Here's how the part is built. I have some questions about the finished solid (model axes, mm). A direction names the side the tool comes from. Give positions to 0.01 mm unless a question says otherwise; leave off trailing zeros. Write each loop counter-clockwise with the first axis right and the second up, starting at its lowest first coordinate (ties: lowest second). Pieces come first, ordered by that corner, then holes. Notation, with made-up numbers: (40, 37) -> (66, 37) arc R23 cw to (66, 65) -> close; hole circle Ø8 at (79, 49.25). An arc over 180 degrees is marked (long way). Put each result on its own line as item: value. Start each with the question number.
from build123d import *

# Parameters (mm, degrees)
SKETCH_W     = 5
SKETCH_H     = 80
PAD_DEPTH    = 61
PAD001_DEPTH = 61
SKETCH002_W  = 49
SKETCH002_H  = 101.034886
POCKET_DEPTH = 19


with BuildPart() as part:
    # Sketch (on YZ_Plane of Origin) → Pad (new body)
    with BuildSketch(Plane.YZ):
        with Locations((-2.5, 40)):
            Rectangle(SKETCH_W, SKETCH_H)
    extrude(amount=PAD_DEPTH)

    # Sketch001 (on Face5 of Pad) → Pad001 (join)
    with BuildSketch(Plane(origin=(0, 0, 0), x_dir=(0, -1, 0), z_dir=(-1, 0, 0))):
        Polygon((0, 0), (0, 36), (0, 40), (-19, 40), (-19, 36), (-13, 36), (-13, 0), align=None)
    extrude(amount=-PAD001_DEPTH)

    # Sketch002 (on Face1 of Pad001) → Pocket (cut)
    with BuildSketch(Plane(origin=(0, 0, 0), x_dir=(-1, 0, 0), z_dir=(0, 1, 0))):
        with Locations((-30.493867, 45)):
            Rectangle(SKETCH002_W, SKETCH002_H)
    extrude(amount=POCKET_DEPTH, mode=Mode.SUBTRACT)


solid = part.part
1) I want a section at A-A, the plane y = 14. Write out the boundary of the cut face in (x, z).
2) I want a section at C-C, the plane z = 30.5. Write out the boundary of the cut face in (x, y), and give its area (3 significant figures).
3) Thinking about a two-plate mould opening in X: for faces 1 (the flat face through (54.994, 7, 20)), 2 (the flat face through (0, 2, 32)), 3 (the flat face through (30, -2, 0)), which applies, released by +X, released by -X, zero draft, split by the parting line, or undercut?
4) I want a section at D-D, the plane z = 68.5. Write out the boundary of the cut face in (x, y), and give its area (3 significant figures).
5) Which directions (+Z, -Z, +X, -X, +Y, -Y) give clear straight access to the entire face, cutting with the end or side of a thin tool? Please do faces 4 (the flat face through (3, 9, 40)), 5 (the flat face through (58, 16, 36)), 6 (the flat face through (5.994, 7, 20)).
6) I need wall thicknesses on probe 1 along X at (y, z) = (15.75, 39.5); probe 2 along Y at (x, z) = (54.5, 60); probe 3 along Z at (x, y) = (3.5, 15.75). Which ranges of each line are inside material? Lowest first, please.
7) I'm going to push flat-ended pins straight in: pin 1 Ø5 at (x, z) = (57, 21) entering from +Y; pin 2 Ø6.5 at (x, y) = (59.5, 6) entering from +Z; pin 3 Ø10 at (x, y) = (47, 12.5) entering from -Z. Where does each tip first touch, or does it pass through?
8) I want a section at B-B, the plane x = 4. Write out the boundary of the cut face in (y, z).
Established:
1. outline: (0, 36) -> (5.99, 36) -> (5.99, 40) -> (0, 40) -> close; (54.99, 36) -> (61, 36) -> (61, 40) -> (54.99, 40) -> close
2. outline: (0, -5) -> (61, -5) -> (61, 13) -> (54.99, 13) -> (54.99, 0) -> (5.99, 0) -> (5.99, 13) -> (0, 13) -> close
2. area: 461 mm2
3. face 1: undercut
3. face 2: released by -X
3. face 3: zero draft
4. outline: (0, -5) -> (61, -5) -> (61, 0) -> (0, 0) -> close
4. area: 305 mm2
5. face 4: +Z, +X, -X, +Y
5. face 5: -Z, +X, -X, +Y
5. face 6: +Z, -Z, +Y
6. probe 1: x = 0 to 5.99, 54.99 to 61
6. probe 2: y = -5 to 0
6. probe 3: z = 36 to 40
7. pin 1: stops at y = 13
7. pin 2: stops at z = 40
7. pin 3: passes through
8. outline: (-5, 0) -> (13, 0) -> (13, 36) -> (19, 36) -> (19, 40) -> (0, 40) -> (0, 80) -> (-5, 80) -> close
